The listing builds one solid part. Answer for the finished solid, in the listing's coordinates (mm). A direction names the side the tool comes from. Round coordinates to 2 decimals unless told otherwise and drop trailing zeros. Order: outer loops, then holes, each group sorted by start corner. A loop starts at its lowest first (then second) coordinate and runs counter-clockwise, first axis right, second up. Notation, with made-up numbers: M 84,35.25 L 133,35.25 A15 cw 133,62.25 Z; hole C 19,18.25 d3. An arc over 180 degrees is marked long. Put each result on its own line as item: value. Start each with the question number.
1. Which of the six approach directions +Z, -Z, +X, -X, +Y, -Y give full straight-line access (tool end or side, diameter ignored) to faces 3 (the face through (9.773, 0, -12)), 4 (the face through (2.29, -23.3, 14.85)), 5 (the face through (7.2, 10, -20.8))?
2. The part is cut by section A-A (y = 0). Count the separate pieces of the cut face and the enclosed holes in it, then the cut area to 3 significant figures.
3. The mould has two halves that part along Z. Classify faces 1 (the face through (7.2, -8.6, -20.3)), 2 (the face through (0, 2, 5)): +Z half, -Z half, draft (parallel to the pull), parting line (faces both ways), or undercut.
4. The part is cut by section C-C (x = 6.5). Give the vertices of the cut face in (y, z).
5. Each of these flat-tipped pins is pushed along its axis until it touches: pin 1 Ø13 at (y, z) = (-11.16, -15.36) entering from +X; pin 2 Ø5 at (x, y) = (4, -7.5) entering from -Z; pin 3 Ø12 at (y, z) = (25, 9.5) entering from +X. Where does it stop, or does it pass through?
6. Consider line 1 (Z direction, x = 7.5, y = 0); line 2 (Y direction, x = 10.75, z = -5.5); line 3 (Y direction, x = 10.75, z = -7). Determine where each line is inside the solid, lowest interval first.
7. The part is cut by section B-B (x = 14.75). Give the vertices of the cut face in (y, z), then the cut area to 3 significant figures.
from build123d import *

# Parameters (mm, degrees)
F2_R     = 5.5659119411
F3_DEPTH = 25
F4_R     = 3
F5_SIZE  = 1


with BuildPart() as f1:
    # F0 (on Front) → F1 (revolve)
    with BuildSketch(Plane.XZ):
        Polygon((0, 11.0889025964), (0, 5.0745825283), (16.1634832621, 5.0745825283), (16.1634832621, 11.0889025964), (9.7732706927, 11.0889025964), (9.7732706927, 27.6282825507), (15.9755358472, 27.6282825507), (15.9755358472, 34.9582345225), (0, 34.9582345225), (0, 27.6282825507), (4.5107388869, 27.6282825507), (4.5107388869, 11.0889025964), align=None)
    revolve(axis=Axis((18.8887231052, 0, 0), (1, 0, 0)))

    # F2 (on face) → F3 (cut)
    with BuildSketch(Plane.YZ.offset(9.7732706927)):
        with Locations((0, 18.9826972783)):
            Circle(F2_R)
        with Locations((18.0536179433, 5.8659760581)):
            Circle(F2_R)
        with Locations((11.1577495089, -15.3573246972)):
            Circle(F2_R)
        with Locations((-18.0536179433, 5.8659760581)):
            Circle(F2_R)
        with Locations((-11.1577495089, -15.3573246972)):
            Circle(F2_R)
    extrude(amount=-F3_DEPTH, mode=Mode.SUBTRACT)

    # F4
    f4_edges = [f1.edges().sort_by_distance(p)[0] for p in [
        (15.975536, 0, -34.958235),
        (0, 0, -34.958235),
    ]]
    fillet(f4_edges, radius=F4_R)

    # F5
    f5_edges = [f1.edges().sort_by_distance(p)[0] for p in [
        (9.773271, 12.487706, 5.865976),
        (9.773271, -5.565912, 18.982697),
        (7.142005, 5.565912, 18.982697),
        (4.510739, -5.565912, 18.982697),
        (9.773271, -23.61953, 5.865976),
        (7.142005, -12.487706, 5.865976),
        (4.510739, -23.61953, 5.865976),
        (9.773271, -16.723661, -15.357325),
        (7.142005, -5.591838, -15.357325),
        (4.510739, -16.723661, -15.357325),
        (9.773271, 5.591838, -15.357325),
        (7.142005, 16.723661, -15.357325),
        (4.510739, 5.591838, -15.357325),
        (7.142005, 23.61953, 5.865976),
        (4.510739, 12.487706, 5.865976),
    ]]
    chamfer(f5_edges, length=F5_SIZE)


solid = f1.part
Resolved:
1. face 3: +X
1. face 4: -X
1. face 5: +X, -X
2. separate pieces: 3
2. enclosed holes: 0
2. area: 534 mm2
3. face 1: undercut
3. face 2: draft
4. outline: C 0,0 d69.92; hole C -18.05,5.87 d11.13; hole C -11.16,-15.36 d11.13; hole C 0,18.98 d11.13; hole C 0,0 d10.15; hole C 11.16,-15.36 d11.13; hole C 18.05,5.87 d11.13
5. pin 1: x = 9.71
5. pin 2: z = -34.6
5. pin 3: x = 15.98
6. line 1: -34.96 to -5.07, 5.07 to 13.42, 24.55 to 34.96
6. line 2: -34.52 to -27.08, -9.63 to 9.63, 27.08 to 34.52
6. line 3: -34.25 to -26.73, -8.6 to 8.6, 26.73 to 34.25
7. outline: C 0,0 d68.75; C 0,0 d22.18; hole C 0,0 d55.26; hole C 0,0 d10.15
7. area: 1,620 mm2
